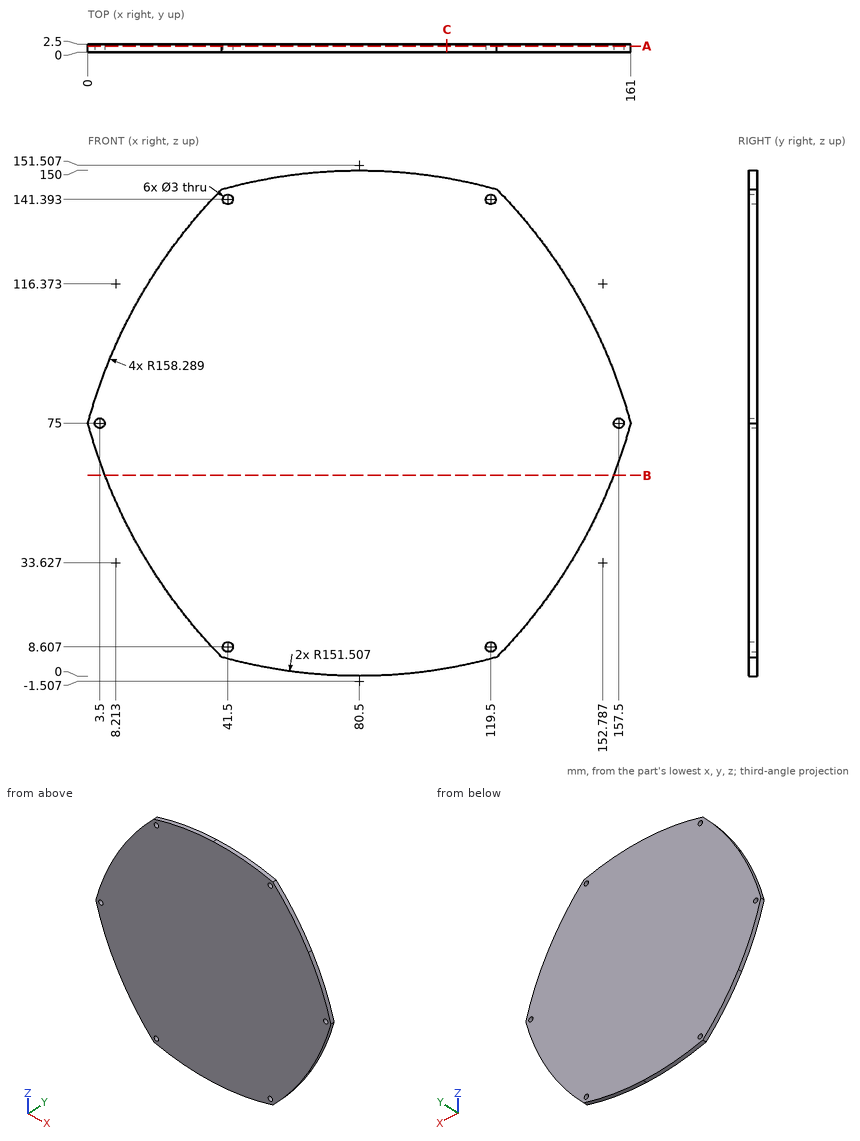
Here's the drawing with two shaded views (mm, measured from the low corner). I have some questions. Coordinates: 2 decimals unless noted, no trailing zeros. Order: outer loops, then holes, each group sorted by start corner. A loop starts at its lowest first (then second) coordinate and runs counter-clockwise, first axis right, second up.
Item 1: If we section it at A-A, the plane y = 1.85: List the corners of the cut face in (x, z) for me (1 decimal), then the cut area to 3 significant figures.
Response values:
outline: (0, 75) arc R158.3 ccw to (39.7, 5.6) arc R151.5 ccw to (121.3, 5.6) arc R158.3 ccw to (161, 75) arc R158.3 ccw to (121.3, 144.4) arc R151.5 ccw to (39.7, 144.4) arc R158.3 ccw to start; hole circle Ø3 at (3.5, 75); hole circle Ø3 at (41.5, 8.6); hole circle Ø3 at (41.5, 141.4); hole circle Ø3 at (119.5, 8.6); hole circle Ø3 at (119.5, 141.4); hole circle Ø3 at (157.5, 75)
area: 18,500 mm2
Item 2: If we section it at C-C, the plane x = 106.5: List the corners of the cut face in (y, z) for me.
Response values:
outline: (0, 2.25) - (2.5, 2.25) - (2.5, 147.75) - (0, 147.75) - close
Item 3: If we section it at B-B, the plane z = 59.5: List the corners of the cut face in (x, y) for me.
Response values:
outline: (5.07, 0) - (155.93, 0) - (155.93, 2.5) - (5.07, 2.5) - close
Item 4: I'm going to push flat-ended pins straight in: pin 1 Ø5 at (x, z) = (41.5, 8.61) entering from +Y; pin 2 Ø1.5 at (y, z) = (2, 25) entering from +X (1 decimal); pin 3 Ø1.5 at (x, y) = (108, 0.5) entering from -Z; pin 4 Ø2.5 at (x, z) = (119.5, 8.61) entering from -Y. Where does each tip first touch, or does it pass through?
Response values:
pin 1: stops at y = 2.5
pin 2: stops at x = 138
pin 3: stops at z = 2.38
pin 4: passes through
Item 5: I need wall thicknesses on probe 1 along X at (y, z) = (0.25, 8.5) (1 decimal); probe 2 along X at (y, z) = (1.8, 44); probe 3 along Z at (x, y) = (56, 0.6) (1 decimal). Which ranges of each line are inside material? Lowest first, please.
Response values:
probe 1: x = 36.9 to 40, 43 to 118, 121 to 124.1
probe 2: x = 12.01 to 148.99
probe 3: z = 2 to 148
